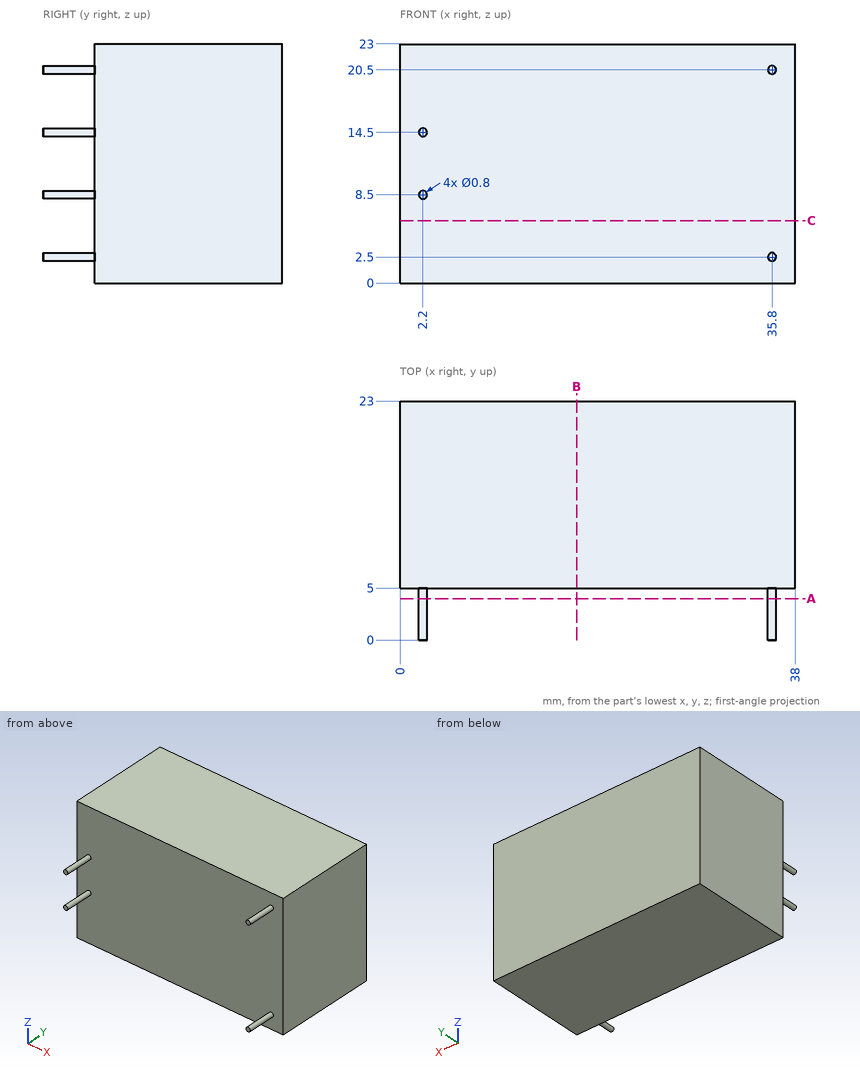
For this review, use the dimensioned drawing (mm, ordinates from the lowest corner) and the shaded views. Round coordinates to 2 decimals unless told otherwise and drop trailing zeros. Order: outer loops, then holes, each group sorted by start corner. A loop starts at its lowest first (then second) coordinate and runs counter-clockwise, first axis right, second up. Notation, with made-up numbers: (-6, -4.75) -> (-1, -4.75) arc R19 ccw to (-1, 32.25) -> close; hole circle Ø1 at (-7, 61). An arc over 180 degrees is marked (long way). Put each result on its own line as item: value.
Q1. Add section B-B on x = 17. Write out the cut boundary in (y, z), plus the area to 3 significant figures.
Check result:
outline: (5, 0) -> (23, 0) -> (23, 23) -> (5, 23) -> close
area: 414 mm2
Q2. Add section A-A on y = 4. Write out the cut boundary in (x, z).
Check result:
outline: circle Ø0.8 at (2.2, 8.5); circle Ø0.8 at (2.2, 14.5); circle Ø0.8 at (35.8, 2.5); circle Ø0.8 at (35.8, 20.5)
Q3. For probe 1 along Y at (x, z) = (18, 13.25); probe 2 along Z at (x, y) = (2, 1), list the stretches that pass through material, from the lowest coordinate up. Write a range as [from, to].
Check result:
probe 1: [5, 23]
probe 2: [8.15, 8.85], [14.15, 14.85]
Q4. Add section C-C on z = 6. Write out the cut boundary in (x, y).
Check result:
outline: (0, 5) -> (38, 5) -> (38, 23) -> (0, 23) -> close
Q5. Insertion check: pin 1 Ø11.5 at (x, z) = (13.5, 7) entering from -Y. The pin has a flat end and moves straight along its axis. Give the tip position at first contact, or say it passes through.
Check result:
pin 1: y = 5
